The model under review builds one solid part; all positions refer to its coordinate system, in mm. A direction names the side the tool comes from. Give positions to 0.01 mm unless a question says otherwise; leave off trailing zeros. Loops run counter-clockwise (first coordinate to the right, second up) from the corner with the lowest first, then second, coordinate; pieces in that order, holes last. Notation, with made-up numbers: M 27.25,-3.5 L 82.25,-3.5 A7 ccw 82.25,4.5 Z; hole C 16,63 d2. An arc over 180 degrees is marked long. Put each result on its own line as item: value. Start each with the question number.
from build123d import *

# Parameters (mm, degrees)
SKETCH_1_R      = 1.75
SKETCH_1_R_2    = 17.5
EXTRUDE_1_DEPTH = 3


with BuildPart() as part:
    # 草图1 → 凸台-拉伸1 (new body)
    with BuildSketch(Plane(origin=(0, 0, 0), x_dir=(1, 0, 0), z_dir=(0, 1, 0))):
        with BuildLine():
            Line((76, 17.5), (68, 17.5))
            Line((68, 17.5), (68, -7))
            Line((68, -7), (76, -7))
            Line((76, -7), (76, -54))
            ThreePointArc((76, -54), (75.121320344, -56.121320344), (73, -57))
            Line((73, -57), (-73, -57))
            ThreePointArc((-73, -57), (-75.121320344, -56.121320344), (-76, -54))
            Line((-76, -54), (-76, 54))
            ThreePointArc((-76, 54), (-75.121320344, 56.121320344), (-73, 57))
            Line((-73, 57), (73, 57))
            ThreePointArc((73, 57), (75.121320344, 56.121320344), (76, 54))
            Line((76, 54), (76, 17.5))
        make_face()
        with Locations(Location((-71, 52, 0), (0, 0, 270))):
            Circle(SKETCH_1_R, mode=Mode.SUBTRACT)
        with Locations(Location((71, 52, 0), (0, 0, 270))):
            Circle(SKETCH_1_R, mode=Mode.SUBTRACT)
        with Locations(Location((71, -52, 0), (0, 0, 270))):
            Circle(SKETCH_1_R, mode=Mode.SUBTRACT)
        with Locations(Location((-71, -52, 0), (0, 0, 270))):
            Circle(SKETCH_1_R, mode=Mode.SUBTRACT)
        with Locations(Location((-4.5, -10.5, 0), (0, 0, 270))):
            Circle(SKETCH_1_R_2, mode=Mode.SUBTRACT)
        with Locations(Location((-20.5, 5.5, 0), (0, 0, 270))):
            Circle(SKETCH_1_R, mode=Mode.SUBTRACT)
        with Locations(Location((11.5, 5.5, 0), (0, 0, 270))):
            Circle(SKETCH_1_R, mode=Mode.SUBTRACT)
        with Locations(Location((11.5, -26.5, 0), (0, 0, 270))):
            Circle(SKETCH_1_R, mode=Mode.SUBTRACT)
        with Locations(Location((-20.5, -26.5, 0), (0, 0, 270))):
            Circle(SKETCH_1_R, mode=Mode.SUBTRACT)
        with Locations(Location((71, 40, 0), (0, 0, 270))):
            Circle(SKETCH_1_R, mode=Mode.SUBTRACT)
        with Locations(Location((22, 40, 0), (0, 0, 270))):
            Circle(SKETCH_1_R, mode=Mode.SUBTRACT)
        with Locations(Location((22, -42, 0), (0, 0, 270))):
            Circle(SKETCH_1_R, mode=Mode.SUBTRACT)
        with Locations(Location((71, -42, 0), (0, 0, 270))):
            Circle(SKETCH_1_R, mode=Mode.SUBTRACT)
        with Locations(Location((-71, 40, 0), (0, 0, 90))):
            Circle(SKETCH_1_R, mode=Mode.SUBTRACT)
        with Locations(Location((-32, 40, 0), (0, 0, 90))):
            Circle(SKETCH_1_R, mode=Mode.SUBTRACT)
        with Locations(Location((-32, -1, 0), (0, 0, 90))):
            Circle(SKETCH_1_R, mode=Mode.SUBTRACT)
        with Locations(Location((-32, -42, 0), (0, 0, 90))):
            Circle(SKETCH_1_R, mode=Mode.SUBTRACT)
        with Locations(Location((-71, -1, 0), (0, 0, 90))):
            Circle(SKETCH_1_R, mode=Mode.SUBTRACT)
        with Locations(Location((-71, -42, 0), (0, 0, 90))):
            Circle(SKETCH_1_R, mode=Mode.SUBTRACT)
    extrude(amount=EXTRUDE_1_DEPTH)


solid = part.part
(1) Insertion check: pin 1 (3 mm diameter, centred on x = 71, z = 42, fed in from -Y). The pin has a flat end and moves straight along its axis. Give the tip position at first contact, or say it passes through.
(2) We need section B-B, the plane z = -52. Write out the cut boundary in (x, y).
(3) We need section C-C, the plane z = 10.5. Write out the cut boundary in (x, y).
(4) We need section A-A, the plane x = -32. Write out the cut boundary in (y, z), plus the area to 4 significant figures.
(5) Draft analysis for pull direction X (two halves, no side actions). For faces 1 (the flat face through (76, 1, -36)), 2 (the flat face through (-1, 1, -57)), 3 (the cylindrical face through (23.5, 1.5, -39.1)), state which applies: +X half, -X half, draft (parallel to the pull), parting line (faces both ways), or undercut.
(6) To check wall thickness, follow L1, parallel to X at y = 1.4, z = 52; L2, parallel to Z at x = -71, y = 1.35; L3, parallel to X at y = 0.2, z = 0. State the ranges of each line that lie inside material, in increasing order. Write a range as [from, to].
(7) For faces 4 (the cylindrical face through (-18.765, 1.479, -5.728)), 5 (the flat face through (72, 1, -17.5)), list the 3-axis set-ups (+Z, -Z, +X, -X, +Y, -Y) from which the entire face can be reached by the end or side of a thin tool; tool diameter is ignored.
(8) We need section D-D, the plane x = -4.5. Write out the cut boundary in (y, z), plus the area to 3 significant figures.
Check sheet entries:
1. pin 1: passes through
2. outline: M -76,0 L -72.75,0 L -72.75,3 L -76,3 Z; M -69.25,0 L 69.25,0 L 69.25,3 L -69.25,3 Z; M 72.75,0 L 76,0 L 76,3 L 72.75,3 Z
3. outline: M -76,0 L -22,0 L -22,3 L -76,3 Z; M 13,0 L 76,0 L 76,3 L 13,3 Z
4. outline: M 0,-57 L 3,-57 L 3,-41.75 L 0,-41.75 Z; M 0,-38.25 L 3,-38.25 L 3,-0.75 L 0,-0.75 Z; M 0,2.75 L 3,2.75 L 3,40.25 L 0,40.25 Z; M 0,43.75 L 3,43.75 L 3,57 L 0,57 Z
4. area: 310.5 mm²
5. face 1: +X half
5. face 2: draft
5. face 3: undercut
6. L1: x = [-76, -72.75], [-69.25, 69.25], [72.75, 76]
6. L2: z = [-57, -53.75], [-50.25, -41.75], [-38.25, -0.75], [2.75, 40.25], [43.75, 50.25], [53.75, 57]
6. L3: x = [-76, -72.44], [-69.56, -33.44], [-30.56, -18.5], [9.5, 68]
7. face 4: +Y, -Y
7. face 5: +X, +Y, -Y
8. outline: M 0,-57 L 3,-57 L 3,-7 L 0,-7 Z; M 0,28 L 3,28 L 3,57 L 0,57 Z
8. area: 237 mm²
